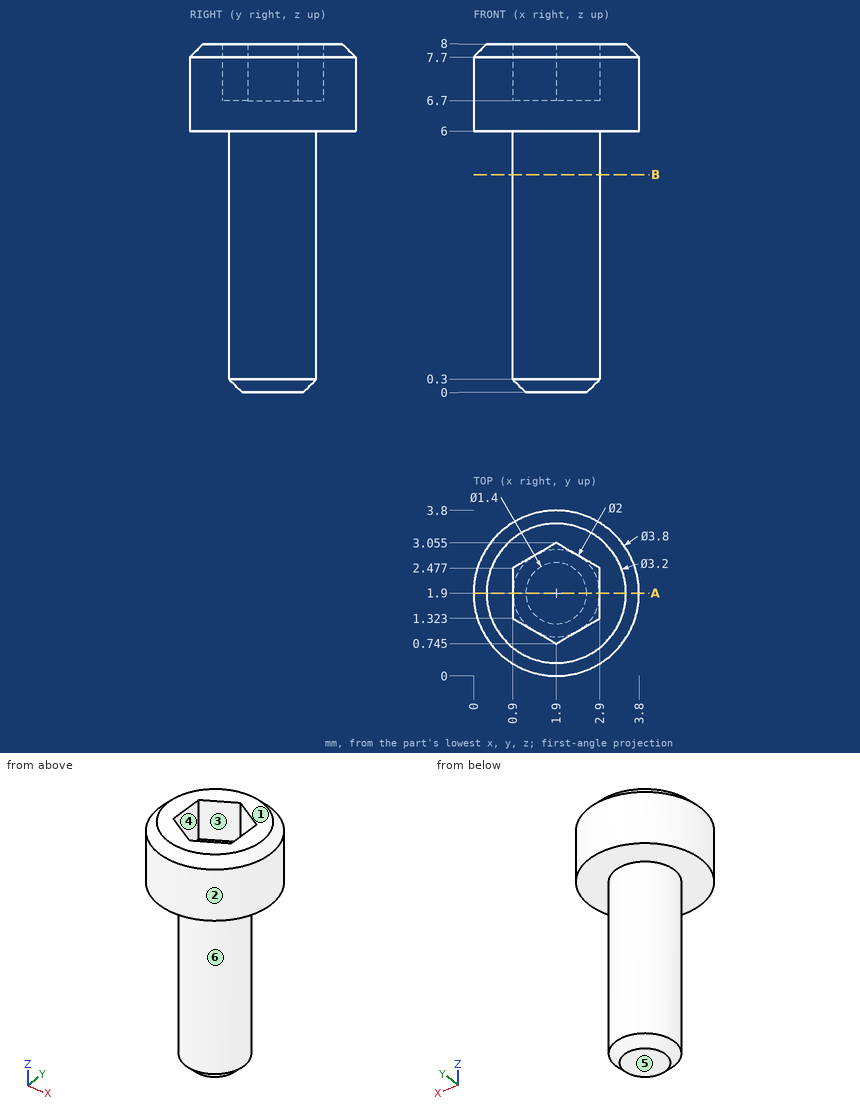
Check sheet for the drawn part. Datum: minimum x, y, z corner. Units: mm. A direction names the side the tool comes from. Round coordinates to 2 decimals unless told otherwise and drop trailing zeros. Order: outer loops, then holes, each group sorted by start corner. A loop starts at its lowest first (then second) coordinate and runs counter-clockwise, first axis right, second up. Notation, with made-up numbers: (58.25, 14) -> (102.25, 14) arc R29 cw to (102.25, 34) -> close; hole circle Ø10 at (55.25, 53). An arc over 180 degrees is marked (long way). Put each result on its own line as item: value.
1) Material ranges on line 1 (Z direction, x = 0.85, y = 2.4); line 2 (X direction, y = 1.85, z = 1); line 3 (Z direction, x = 1.85, y = 2.55), recorded low to high.
Final values:
line 1: z = 6 to 8
line 2: x = 0.9 to 2.9
line 3: z = 0 to 6.7
2) Set-up check for the marked faces 4, 5 and 6: record each of +Z, -Z, +X, -X, +Y, -Y from which the full face is reachable in a straight line by a thin tool's end or side.
Final values:
face 4: +Z
face 5: -Z, +X, -X, +Y, -Y
face 6: -Z
3) Depth check by flat-ended pin: pin 1 (1.5 mm diameter, centred on x = 1, y = 3.5, fed in from -Z); pin 2 (0.6 mm diameter, centred on x = 2, y = 2.5, fed in from +Z); pin 3 (1.5 mm diameter, centred on x = 3, z = 3.5, fed in from -Y). Enter the tip coordinate at first touch or a pass-through.
Final values:
pin 1: stops at z = 6
pin 2: stops at z = 6.7
pin 3: stops at y = 0.96
4) Section check B-B (z = 5). Record the cut outline in (x, y).
Final values:
outline: circle Ø2 at (1.9, 1.9)
5) Section check A-A (y = 1.9). Record the cut outline in (x, z).
Final values:
outline: (0, 6) -> (0.9, 6) -> (0.9, 0.3) -> (1.2, 0) -> (2.6, 0) -> (2.9, 0.3) -> (2.9, 6) -> (3.8, 6) -> (3.8, 7.7) -> (3.5, 8) -> (2.9, 8) -> (2.9, 6.7) -> (0.9, 6.7) -> (0.9, 8) -> (0.3, 8) -> (0, 7.7) -> close
6) Mould release check, pull along Y, two halves, no side actions. Record for the marked faces 1, 2 and 3: +Y half, -Y half, draft (parallel to the pull), parting line (faces both ways), or undercut.
Final values:
face 1: draft
face 2: parting line
face 3: undercut
